Verification items for the finished model (mm, model axes). A direction names the side the tool comes from. Coordinates: 2 decimals unless noted, no trailing zeros. Write each loop counter-clockwise with the first axis right and the second up, starting at its lowest first coordinate (ties: lowest second). Pieces come first, ordered by that corner, then holes. Notation, with made-up numbers: (54.25, -12.75) -> (65.25, -12.75) arc R36 cw to (65.25, 21.25) -> close; hole circle Ø8 at (29, -9.75). An arc over 180 degrees is marked (long way). Write each question's results on one line, items separated by ' | '. Start each with the question number.
Autodesk Inventor part; units mm, degrees
ref_plane "YZ Plane" through (0, 0, 0) normal (1, 0, 0) x (0, 1, 0)
ref_plane "XZ Plane" through (0, 0, 0) normal (0, 1, 0) x (-1, 0, 0)
ref_plane "XY Plane" through (0, 0, 0) normal (0, 0, 1) x (1, 0, 0)
sketch "Sketch1" plane through (0, 0, 0) normal (0, 0, 1) x (1, 0, 0)
  circle A0 centre (0, 0) radius 6.5
  line L0 (0, 0) -> (16, 0) construction
  arc A1 (10.1847, 0.9) -> (6.1847, 2) centre (4.2455, -12.8741) ccw
  arc A2 (6.1847, -2) -> (10.1847, -0.9) centre (4.2455, 12.8741) ccw
  arc A3 (6.1847, -2) -> (6.1847, 2) centre (0, 0) ccw
  arc A4 (10.1847, -0.9) -> (10.1847, 0.9) centre (-9.7951, 0) ccw
  arc A5 (7.2234, 7.236) -> (3.4521, 5.5075) centre (11.5276, -7.1332) ccw
  arc A6 (8.3804, 5.8571) -> (7.2234, 7.236) centre (-7.5035, -6.2962) ccw
  arc A7 (6.0233, 2.4433) -> (8.3804, 5.8571) centre (-5.0231, 12.5911) ccw
  arc A8 (6.0233, 2.4433) -> (3.4521, 5.5075) centre (0, 0) ccw
  arc A9 (0.8822, 10.1862) -> (-0.8957, 6.438) centre (13.4158, 1.9455) ccw
  arc A10 (2.6549, 9.8736) -> (0.8822, 10.1862) centre (-1.7009, -9.6463) ccw
  arc A11 (3.0436, 5.7434) -> (2.6549, 9.8736) centre (-11.9413, 6.4166) ccw
  arc A12 (3.0436, 5.7434) -> (-0.8957, 6.438) centre (0, 0) ccw
  arc A13 (-5.8718, 8.3702) -> (-4.8244, 4.3561) centre (9.0266, 10.1138) ccw
  arc A14 (-4.3129, 9.2702) -> (-5.8718, 8.3702) centre (4.8975, -8.4828) ccw
  arc A15 (-1.3603, 6.3561) -> (-4.3129, 9.2702) centre (-13.2721, -2.7603) ccw
  arc A16 (-1.3603, 6.3561) -> (-4.8244, 4.3561) centre (0, 0) ccw
  arc A17 (-9.8783, 2.6376) -> (-6.4957, 0.2359) centre (0.4137, 13.5498) ccw
  arc A18 (-9.2626, 4.3291) -> (-9.8783, 2.6376) centre (9.2044, -3.3501) ccw
  arc A19 (-5.1276, 3.9947) -> (-9.2626, 4.3291) centre (-8.3927, -10.6457) ccw
  arc A20 (-5.1276, 3.9947) -> (-6.4957, 0.2359) centre (0, 0) ccw
  arc A21 (-9.2626, -4.3291) -> (-5.1276, -3.9947) centre (-8.3927, 10.6457) ccw
  arc A22 (-9.8783, -2.6376) -> (-9.2626, -4.3291) centre (9.2044, 3.3501) ccw
  arc A23 (-6.4957, -0.2359) -> (-9.8783, -2.6376) centre (0.4137, -13.5498) ccw
  arc A24 (-6.4957, -0.2359) -> (-5.1276, -3.9947) centre (0, 0) ccw
  arc A25 (-4.3129, -9.2702) -> (-1.3603, -6.3561) centre (-13.2721, 2.7603) ccw
  arc A26 (-5.8718, -8.3702) -> (-4.3129, -9.2702) centre (4.8975, 8.4828) ccw
  arc A27 (-4.8244, -4.3561) -> (-5.8718, -8.3702) centre (9.0266, -10.1138) ccw
  arc A28 (-4.8244, -4.3561) -> (-1.3603, -6.3561) centre (0, 0) ccw
  arc A29 (2.6549, -9.8736) -> (3.0436, -5.7434) centre (-11.9413, -6.4166) ccw
  arc A30 (0.8822, -10.1862) -> (2.6549, -9.8736) centre (-1.7009, 9.6463) ccw
  arc A31 (-0.8957, -6.438) -> (0.8822, -10.1862) centre (13.4158, -1.9455) ccw
  arc A32 (-0.8957, -6.438) -> (3.0436, -5.7434) centre (0, 0) ccw
  arc A33 (8.3804, -5.8571) -> (6.0233, -2.4433) centre (-5.0231, -12.5911) ccw
  arc A34 (7.2234, -7.236) -> (8.3804, -5.8571) centre (-7.5035, 6.2962) ccw
  arc A35 (3.4521, -5.5075) -> (7.2234, -7.236) centre (11.5276, 7.1332) ccw
  arc A36 (3.4521, -5.5075) -> (6.0233, -2.4433) centre (0, 0) ccw
  point P0 (10.2049, 0)
  point P1 (7.8174, 6.5596)
  point P2 (1.7721, 10.0499)
  point P3 (-5.1025, 8.8377)
  point P4 (-9.5895, 3.4903)
  point P5 (-9.5895, -3.4903)
  point P6 (-5.1025, -8.8377)
  point P7 (1.7721, -10.0499)
  point P8 (7.8174, -6.5596)
  dimension "d0" = 13
  dimension "d1" = 16
  dimension "d2" = 15
  dimension "d3" = 4
  dimension "d4" = 2
  dimension "d6" = 1.8
  dimension "d15" = 20
  dimension "d18" = 360
extrude "Extrusion1" add sketch "Sketch1" along normal blind 10
sketch "Sketch5" plane through (0, 0, 10) normal (0, 0, 1) x (1, 0, 0)
  circle A0 centre (0, 0) radius 2.75
  dimension "d32" = 5.5
extrude "Extrusion5" cut sketch "Sketch5" against normal through all
properties part number "Motor Gear" material "ABS Plastic"
1. Sectioned sample at B-B on y = -7.75. Record the cut outline in (x, z), plus the area to 3 significant figures.
2. Sectioned sample at C-C on x = 4.5. Record the cut outline in (y, z).
3. Material ranges on probe 1 along Y at (x, z) = (7.75, 2.75); probe 2 along Y at (x, z) = (2, 8); probe 3 along X at (y, z) = (6.75, 1), recorded low to high. Write a range as from..to.
4. Sectioned sample at D-D on y = 3. Record the cut outline in (x, z), plus the area to 3 significant figures.
5. Mould release check, pull along Y, two halves, no side actions. Record for faces 1 (the cylindrical face through (-0.15, 8.35, 4.93)), 2 (the cylindrical face through (-7.213, 4.308, 4.93)), 3 (the cylindrical face through (8.25, -1.58, 4.93)): +Y half, -Y half, draft (parallel to the pull), parting line (faces both ways), or undercut.
6. Depth check by flat-ended pin: pin 1 Ø1.5 at (y, z) = (-7.5, 6.5) entering from -X. Enter the tip coordinate at first touch or a pass-through.
7. Sectioned sample at A-A on x = -6.75. Record the cut outline in (y, z), plus the area to 3 significant figures.
8. Tool access check on faces 4 (the cylindrical face through (5.25, 6.49, 4.93)), 5 (the cylindrical face through (-2.715, -7.895, 4.93)), 6 (the cylindrical face through (7.337, 4.092, 4.93)), 7 (the cylindrical face through (1.76, 10.05, 4.93)). Record the directions out of +Z, -Z, +X, -X, +Y, -Y that give a thin tool (end or side, any length) a straight path to the whole face; none if there is none.
Computed values:
1) outline: (-5.79, 0) -> (-2.57, 0) -> (-2.57, 10) -> (-5.79, 10) -> close; (-0.42, 0) -> (3, 0) -> (3, 10) -> (-0.42, 10) -> close | area: 66.3 mm^2
2) outline: (-6.12, 0) -> (6.12, 0) -> (6.12, 10) -> (-6.12, 10) -> close
3) probe 1: y = -6.64..-4.73, -1.71..1.71, 4.73..6.64 | probe 2: y = -10.01..-1.89, 1.89..10.01 | probe 3: x = -5.59..-1.67, -0.79..3.06, 5.85..7.66
4) outline: (-9.76, 0) -> (6.51, 0) -> (6.51, 10) -> (-9.76, 10) -> close | area: 163 mm^2
5) face 1: +Y half | face 2: undercut | face 3: undercut
6) pin 1: stops at x = -5.86
7) outline: (-4.26, 0) -> (-0.37, 0) -> (-0.37, 10) -> (-4.26, 10) -> close; (0.37, 0) -> (4.26, 0) -> (4.26, 10) -> (0.37, 10) -> close | area: 77.9 mm^2
8) face 4: +Z, -Z, +Y | face 5: +Z, -Z, -Y | face 6: +Z, -Z, +X | face 7: +Z, -Z, +X, +Y
